Geometry check sheet. Reference: the model listing, model coordinates, mm. A direction names the side the tool comes from. Round coordinates to 2 decimals unless told otherwise and drop trailing zeros. Order: outer loops, then holes, each group sorted by start corner. A loop starts at its lowest first (then second) coordinate and runs counter-clockwise, first axis right, second up. Notation, with made-up numbers: M 63,86 L 99,86 A16 ccw 99,98 Z; hole C 48.25,22.25 d6. An arc over 180 degrees is marked long. Answer as a JSON object with one key per item and string values. Group by question number.
```python
from build123d import *

# Parameters (mm, degrees)
F1_DEPTH = 10


with BuildPart() as f1:
    # F0 (on Front) → F1 (new body)
    with BuildSketch(Plane.XZ):
        Polygon((2.5655252267, -7.8958747543), (4.8799189691, -6.7166322424), (6.7166322424, -4.8799189691), (7.8958747543, -2.5655252267), (8.3022140315, 0), (7.8958747543, 2.5655252267), (6.7166322424, 4.8799189691), (4.8799189691, 6.7166322424), (2.5655252267, 7.8958747543), (0, 8.3022140315), (-2.5655252267, 7.8958747543), (-4.8799189691, 6.7166322424), (-6.7166322424, 4.8799189691), (-7.8958747543, 2.5655252267), (-8.3022140315, 0), (-7.8958747543, -2.5655252267), (-6.7166322424, -4.8799189691), (-4.8799189691, -6.7166322424), (-2.5655252267, -7.8958747543), (0, -8.3022140315), align=None)
        Polygon((0.1586110624, 3.9968540793), (1.2293142469, 3.7834402195), (1.385943919, 3.752220603), (2.4776109283, 3.1402936308), (3.3267521175, 2.2209728384), (3.8502476305, 1.0842477501), (3.9968540793, -0.1586110624), (3.752220603, -1.385943919), (3.1402936308, -2.4776109283), (2.2209728384, -3.3267521175), (1.0842477501, -3.8502476305), (-0.1586110624, -3.9968540793), (-1.385943919, -3.752220603), (-2.4776109283, -3.1402936308), (-3.3267521175, -2.2209728384), (-3.8502476305, -1.0842477501), (-3.9968540793, 0.1586110624), (-3.752220603, 1.385943919), (-3.1402936308, 2.4776109283), (-2.2209728384, 3.3267521175), (-1.0842477501, 3.8502476305), align=None, mode=Mode.SUBTRACT)
        Polygon((-6.3492907419, 6.3078528102), (-6.7166322424, 4.8799189691), (-4.8799189691, 6.7166322424), align=None)
        Polygon((-4.8799189691, 6.7166322424), (-2.5655252267, 7.8958747543), (-4.0893006175, 7.9611632604), align=None)
        Polygon((-2.5655252267, 7.8958747543), (0, 8.3022140315), (-1.4290212569, 8.8351795821), align=None)
        Polygon((0, 8.3022140315), (2.5655252267, 7.8958747543), (1.3711406609, 8.8443469679), align=None)
        Polygon((2.5655252267, 7.8958747543), (4.8799189691, 6.7166322424), (4.0370857775, 7.9877680503), align=None)
        Polygon((4.8799189691, 6.7166322424), (6.7166322424, 4.8799189691), (6.3078528102, 6.3492907419), align=None)
        Polygon((6.7166322424, 4.8799189691), (7.8958747543, 2.5655252267), (7.9611632604, 4.0893006175), align=None)
        Polygon((7.8958747543, 2.5655252267), (8.3022140315, 0), (8.8351795821, 1.4290212569), align=None)
        Polygon((8.3022140315, 0), (7.8958747543, -2.5655252267), (8.8443469679, -1.3711406609), align=None)
        Polygon((7.8958747543, -2.5655252267), (6.7166322424, -4.8799189691), (7.9877680503, -4.0370857775), align=None)
        Polygon((6.7166322424, -4.8799189691), (4.8799189691, -6.7166322424), (6.3492907419, -6.3078528102), align=None)
        Polygon((4.0893006175, -7.9611632604), (4.8799189691, -6.7166322424), (2.5655252267, -7.8958747543), align=None)
        Polygon((1.4290212569, -8.8351795821), (2.5655252267, -7.8958747543), (0, -8.3022140315), align=None)
        Polygon((-1.3711406609, -8.8443469679), (0, -8.3022140315), (-2.5655252267, -7.8958747543), align=None)
        Polygon((-4.0370857775, -7.9877680503), (-2.5655252267, -7.8958747543), (-4.8799189691, -6.7166322424), align=None)
        Polygon((-6.3078528102, -6.3492907419), (-4.8799189691, -6.7166322424), (-6.7166322424, -4.8799189691), align=None)
        Polygon((-7.9611632604, -4.0893006175), (-6.7166322424, -4.8799189691), (-7.8958747543, -2.5655252267), align=None)
        Polygon((-8.8351795821, -1.4290212569), (-7.8958747543, -2.5655252267), (-8.3022140315, 0), align=None)
        Polygon((-7.9877680503, 4.0370857775), (-7.8958747543, 2.5655252267), (-6.7166322424, 4.8799189691), align=None)
        Polygon((-8.8443469679, 1.3711406609), (-8.3022140315, 0), (-7.8958747543, 2.5655252267), align=None)
        Polygon((-1.760271545, -3.1402936308), (-2.4776109283, -3.1402936308), (-1.385943919, -3.752220603), align=None)
        Polygon((-0.7037136241, -3.5305505428), (-1.385943919, -3.752220603), (-0.1586110624, -3.9968540793), align=None)
        Polygon((-0.1586110624, -3.9968540793), (1.0842477501, -3.8502476305), (0.4217286894, -3.5752125689), align=None)
        Polygon((1.0842477501, -3.8502476305), (2.2209728384, -3.3267521175), (1.5058892605, -3.2699078787), align=None)
        Polygon((2.2209728384, -3.3267521175), (3.1402936308, -2.4776109283), (2.4426428986, -2.6445218226), align=None)
        Polygon((3.1402936308, -2.4776109283), (3.752220603, -1.385943919), (3.1402936308, -1.760271545), align=None)
        Polygon((3.752220603, -1.385943919), (3.9968540793, -0.1586110624), (3.5305505428, -0.7037136241), align=None)
        Polygon((3.9968540793, -0.1586110624), (3.8502476305, 1.0842477501), (3.5752125689, 0.4217286894), align=None)
        Polygon((3.8502476305, 1.0842477501), (3.3267521175, 2.2209728384), (3.2699078787, 1.5058892605), align=None)
        Polygon((3.3267521175, 2.2209728384), (2.4776109283, 3.1402936308), (2.6445218226, 2.4426428986), align=None)
        Polygon((2.4776109283, 3.1402936308), (1.385943919, 3.752220603), (1.760271545, 3.1402936308), align=None)
        Polygon((-3.2699078787, -1.5058892605), (-3.8502476305, -1.0842477501), (-3.3267521175, -2.2209728384), align=None)
        Polygon((-2.4426428986, 2.6445218226), (-2.2209728384, 3.3267521175), (-3.1402936308, 2.4776109283), align=None)
        Polygon((-1.5058892605, 3.2699078787), (-1.0842477501, 3.8502476305), (-2.2209728384, 3.3267521175), align=None)
        Polygon((-0.4217286894, 3.5752125689), (0.1586110624, 3.9968540793), (-1.0842477501, 3.8502476305), align=None)
        Polygon((-3.1402936308, 1.760271545), (-3.1402936308, 2.4776109283), (-3.752220603, 1.385943919), align=None)
        Polygon((-3.5305505428, 0.7037136241), (-3.752220603, 1.385943919), (-3.9968540793, 0.1586110624), align=None)
        Polygon((-3.5752125689, -0.4217286894), (-3.9968540793, 0.1586110624), (-3.8502476305, -1.0842477501), align=None)
        Polygon((-2.6445218226, -2.4426428986), (-3.3267521175, -2.2209728384), (-2.4776109283, -3.1402936308), align=None)
        Polygon((1.1994854323, 3.6916365681), (1.2293142469, 3.7834402195), (0.1586110624, 3.9968540793), (0.7037136241, 3.5305505428), align=None)
    extrude(amount=F1_DEPTH)


solid = f1.part
```
1) Set-up check for faces 5 (the flat face through (-3.32, -4.93, 7.93)), 6 (the flat face through (-0.7, -4.93, -8.58)), 7 (the flat face through (-7.348, -4.93, -4.479)): record each of +Z, -Z, +X, -X, +Y, -Y from which the full face is reachable in a straight line by a thin tool's end or side.
2) Sectioned sample at B-B (x = -7.5). Record the boundary of the cut face in (y, z).
3) Go/stop test with flat-tipped pins: P1, Ø3, axis at y = -6, z = 3.5, coming from the -X side; P2, Ø5, axis at y = -6, z = 4.5, coming from the +X side; P3, Ø2, axis at y = -7.5, z = 7, coming from the +X side (3 decimals). Record where each tip stops, or that it passes through.
4) Release check for a two-part mould opening along Z. For faces 1 (the flat face through (-5.604, -4.93, 6.515)), 2 (the flat face through (1.99, -4.93, -8.37)), 3 (the flat face through (4, -10, -2)), 4 (the flat face through (8.58, -4.93, -0.7)) record: +Z half, -Z half, draft (parallel to the pull), parting line (faces both ways), or undercut.
5) Sectioned sample at A-A (z = -7.25). Record the boundary of the cut face in (x, y), then the cut area to 3 significant figures.
6) Thickness scan on line 1 along X through (y, z) = (-8.25, -2); line 2 along X through (y, z) = (-7.5, -1); line 3 along Z through (x, y) = (-0.25, -3.5). Record the ranges inside material, lowest first. Write a range as [from, to].
Final values:
{
 "1": {"face 5": "+Z, +Y, -Y", "face 6": "-Z, +Y, -Y", "face 7": "-Z, -X, +Y, -Y"},
 "2": {"outline": "M -10,-4.38 L 0,-4.38 L 0,4.36 L -10,4.36 Z"},
 "3": {"P1": "stops at x = -8.34", "P2": "stops at x = 8.36", "P3": "stops at x = 6.405"},
 "4": {"face 1": "+Z half", "face 2": "-Z half", "face 3": "draft", "face 4": "undercut"},
 "5": {"outline": "M -4.53,-10 L 4.54,-10 L 4.54,0 L -4.53,0 Z", "area": "90.7 mm^2"},
 "6": {"line 1": "x = [-8.36, -3.31], [3.14, 8.34]", "line 2": "x = [-8.68, -3.82], [3.63, 8.7]", "line 3": "z = [-8.4, -3.92], [3.7, 8.4]"}
}
